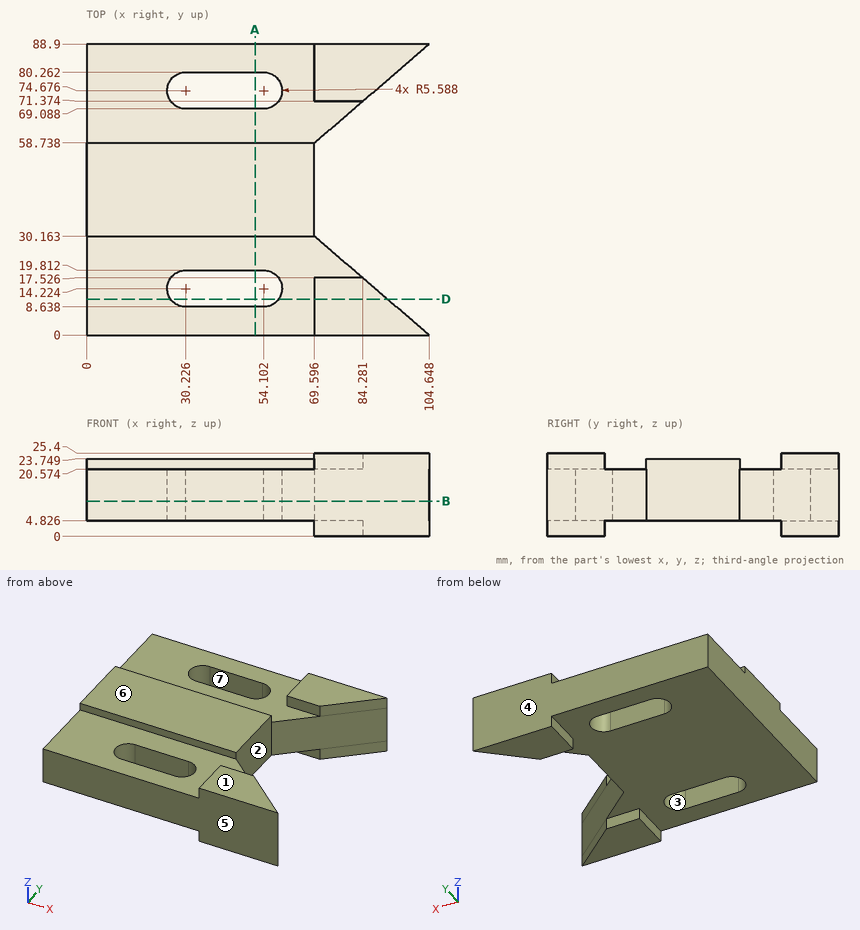
Geometry check sheet. Reference: drawing and pictorial views, mm from the part's lowest x, y, z. A direction names the side the tool comes from. Give positions to 0.01 mm unless a question says otherwise; leave off trailing zeros. Loops run counter-clockwise (first coordinate to the right, second up) from the corner with the lowest first, then second, coordinate; pieces in that order, holes last. Notation, with made-up numbers: M 71,36 L 86,36 A25 ccw 86,54 Z; hole C 23,-5 d11. An arc over 180 degrees is marked long. One line per question, with ' | ' between items.
Item 1: Section check D-D, the plane y = 11. Record the cut outline in (x, z) (1 decimal), plus the area to 3 significant figures.
Completed:
outline: M 0,4.8 L 25.7,4.8 L 25.7,20.6 L 0,20.6 Z; M 58.7,4.8 L 69.6,4.8 L 69.6,0 L 91.9,0 L 91.9,25.4 L 69.6,25.4 L 69.6,20.6 L 58.7,20.6 Z | area: 1,140 mm^2
Item 2: Section check A-A, the plane x = 51.5. State how many separate pieces and enclosed holes the cut face has, plus the area to 3 significant figures.
Completed:
separate pieces: 3 | enclosed holes: 0 | area: 1,140 mm^2
Item 3: Section check B-B, the plane z = 10.75. Record the cut outline in (x, y) (1 decimal).
Completed:
outline: M 0,0 L 104.6,0 L 69.6,30.2 L 69.6,58.7 L 104.6,88.9 L 0,88.9 Z; hole M 30.2,19.8 A5.6 ccw long 30.4,8.6 L 54,8.6 A5.6 ccw long 54.1,19.8 Z; hole M 30.2,69.1 L 54.1,69.1 A5.6 ccw long 54,80.3 L 30.4,80.3 A5.6 ccw long Z
Item 4: Draft check along Y on the marked faces 4, 5, 6 and 7. Enter one of: +Y half, -Y half, draft (parallel to the pull), parting line (faces both ways), or undercut.
Completed:
face 4: +Y half | face 5: -Y half | face 6: draft | face 7: undercut
Item 5: Depth check by flat-ended pin: P1, Ø8.5, axis at x = 23.5, y = 41.5, coming from the +Z side; P2, Ø5, axis at x = 36.5, z = 3.5, coming from the +Y side; P3, Ø5.5, axis at y = 10, z = 24, coming from the -X side; P4, Ø2.5, axis at x = 44, z = 22, coming from the -Y side. Enter the tip coordinate at first touch or a pass-through.
Completed:
P1: stops at z = 23.75 | P2: stops at y = 88.9 | P3: stops at x = 69.6 | P4: stops at y = 30.16
Item 6: Thickness scan on line 1 (Y direction, x = 50.5, z = 9.5); line 2 (Y direction, x = 84, z = 21.5) (1 decimal); line 3 (Y direction, x = 25.5, z = 11.5) (1 decimal). Record the ranges inside material, lowest first. Write a range as [from, to].
Completed:
line 1: y = [0, 8.64], [19.81, 69.09], [80.26, 88.9] | line 2: y = [0, 17.5], [71.4, 88.9] | line 3: y = [0, 11.2], [17.2, 71.7], [77.7, 88.9]
Item 7: Tool access check on the marked faces 1, 2 and 3. Record the directions out of +Z, -Z, +X, -X, +Y, -Y that give a thin tool (end or side, any length) a straight path to the whole face; none if there is none.
Completed:
face 1: +Z, +X, -X, +Y, -Y | face 2: +Z, -Z, +X | face 3: +Z, -Z
